```python
from build123d import *

# Parameters (mm, degrees)
CUT_EXTRUDE1_DEPTH   = 4.953
MIRROR2_COPY_1_DEPTH = 4.953
LPATTERN1_COUNT      = 4
LPATTERN1_PITCH      = 4.92125
SKETCH5_R            = 4.7625
CUT_EXTRUDE2_DEPTH   = 24.60625


with BuildPart() as part:
    # Sketch2 → Revolve1 (revolve)
    with BuildSketch(Plane(origin=(0, 0, 0), x_dir=(0, 0, -1), z_dir=(1, 0, 0))):
        Polygon((-55.5625, 0), (-55.5625, 7.46125), (-30.95625, 7.46125), (-30.95625, 14.2875), (30.95625, 14.2875), (30.95625, 7.46125), (55.5625, 7.46125), (55.5625, 0), align=None)
    revolve(axis=Axis((0, 0, -30.95625), (0, 0, 1)))

    # Sketch3 → Cut-Extrude1 (cut)
    with BuildSketch(Plane(origin=(0, 0, -30.95625), x_dir=(-1, 0, 0), z_dir=(0, 0, -1))):
        with BuildLine():
            Line((-8.5725, 11.43), (8.5725, 11.43))
            ThreePointArc((8.5725, 11.43), (0, 14.2875), (-8.5725, 11.43))
        make_face()
    cut_extrude1 = extrude(amount=-CUT_EXTRUDE1_DEPTH, mode=Mode.SUBTRACT)

    # Mirror1: Cut-Extrude1 across plane
    add(cut_extrude1.mirror(Plane.ZX), mode=Mode.SUBTRACT)

    # Mirror2: Cut-Extrude1 across plane
    add(cut_extrude1.mirror(Plane.XY), mode=Mode.SUBTRACT)

    # Mirror2 copy 1 sketch → Mirror2 copy 1 (cut)
    with BuildSketch(Plane(origin=(0, 0, 30.95625), x_dir=(-1, 0, 0), z_dir=(0, 0, 1))):
        with BuildLine():
            Line((-8.5725, 11.43), (8.5725, 11.43))
            ThreePointArc((8.5725, 11.43), (0, 14.2875), (-8.5725, 11.43))
        make_face()
    extrude(amount=-MIRROR2_COPY_1_DEPTH, mode=Mode.SUBTRACT)

    # Sketch4 → Cut-Revolve1 (revolve, cut)
    with BuildSketch(Plane(origin=(0, 0, 0), x_dir=(0, 0, -1), z_dir=(1, 0, 0))):
        Polygon((-55.5625, 7.46125), (-55.5625, 6.35), (-50.64125, 7.46125), align=None)
    cut_revolve1 = revolve(axis=Axis((0, 0, -55.5625), (0, 0, 1)), mode=Mode.SUBTRACT)

    # LPattern1: Cut-Revolve1 ×4
    with Locations(*[(0, 0, -i * LPATTERN1_PITCH) for i in range(1, LPATTERN1_COUNT)]):
        add(cut_revolve1, mode=Mode.SUBTRACT)

    # Mirror3: Cut-Revolve1 across plane
    add(cut_revolve1.mirror(Plane.XY), mode=Mode.SUBTRACT)

    # Mirror3 copy 1 sketch → Mirror3 copy 1 (revolve, cut)
    with BuildSketch(Plane(origin=(0, 0, 4.92125), x_dir=(0, 0, 1), z_dir=(1, 0, 0))):
        Polygon((-55.5625, -7.46125), (-55.5625, -6.35), (-50.64125, -7.46125), align=None)
    revolve(axis=Axis((0, 0, 60.48375), (0, 0, 1)), mode=Mode.SUBTRACT)

    # Mirror3 copy 2 sketch → Mirror3 copy 2 (revolve, cut)
    with BuildSketch(Plane(origin=(0, 0, 9.8425), x_dir=(0, 0, 1), z_dir=(1, 0, 0))):
        Polygon((-55.5625, -7.46125), (-55.5625, -6.35), (-50.64125, -7.46125), align=None)
    revolve(axis=Axis((0, 0, 65.405), (0, 0, 1)), mode=Mode.SUBTRACT)

    # Mirror3 copy 3 sketch → Mirror3 copy 3 (revolve, cut)
    with BuildSketch(Plane(origin=(0, 0, 14.76375), x_dir=(0, 0, 1), z_dir=(1, 0, 0))):
        Polygon((-55.5625, -7.46125), (-55.5625, -6.35), (-50.64125, -7.46125), align=None)
    revolve(axis=Axis((0, 0, 70.32625), (0, 0, 1)), mode=Mode.SUBTRACT)

    # Sketch5 → Cut-Extrude2 (cut)
    with BuildSketch(Plane.XY.offset(55.5625)):
        Circle(SKETCH5_R)
    cut_extrude2 = extrude(amount=-CUT_EXTRUDE2_DEPTH, mode=Mode.SUBTRACT)

    # Mirror4: Cut-Extrude2 across plane
    add(cut_extrude2.mirror(Plane.XY), mode=Mode.SUBTRACT)


solid = part.part
```
The listing builds one solid part. Answer for the finished solid, in the listing's coordinates (mm). A direction names the side the tool comes from. Coordinates: 2 decimals unless noted, no trailing zeros. Write each loop counter-clockwise with the first axis right and the second up, starting at its lowest first coordinate (ties: lowest second). Pieces come first, ordered by that corner, then holes. Notation, with made-up numbers: M -26.75,-23 L 32.25,-23 A30 cw 32.25,13 Z; hole C -10.75,47 d10. An arc over 180 degrees is marked long. Use a Markdown table: item, result. Add a question column.
1. Section B-B (z = -14) is taken. Give the vertices of the cut face in (x, y) (1 decimal), plus the area to 3 significant figures.
2. For a pull along X with two mould halves and no side action, classify faces 5 (the flat face through (0, -8, -30.956)), 6 (the flat face through (0, 0, 30.956)), 7 (the conical face through (6.387, -1.418, -54.708)) as +X half, -X half, draft (parallel to the pull), parting line (faces both ways), or undercut.
3. Section C-C (y = 8.5) is taken. Give the vertices of the cut face in (x, z), plus the area to 3 significant figures.
4. Straight lines are drawn through the part: line 1 along Z through (x, y) = (10, 4); line 2 along Z through (x, y) = (3, -12.25); line 3 along Y through (x, z) = (0, 44.75). For each, find the intervals that lie inside material, in ascending order. Write a range as [from, to].
5. Section A-A (z = 34) is taken. Give the vertices of the cut face in (x, y) (1 decimal), plus the area to 3 significant figures.
6. Given P1, Ø1.5, axis at x = 2.5, z = 29.5, coming from the -Y side; P2, Ø4, axis at y = -10, z = 1.5, coming from the -X side; P3, Ø2.5, axis at x = 0.5, y = 12.5, coming from the +Z side; P4, Ø2, axis at y = 10, z = -32.5, coming from the +X side, each flat-ended and moving along its own axis, determine where each tip first touches the part or whether it passes through.
7. Which of the six approach directions +Z, -Z, +X, -X, +Y, -Y give full straight-line access (tool end or side, diameter ignored) to faces 1 (the flat face through (0, -13, -26.003)), 2 (the cylindrical face through (-3.78, -2.9, -43.43)), 3 (the conical face through (6.387, -1.418, -44.865)), 4 (the flat face through (0, 13, 26.003))?
8. Section D-D (x = -11.5) is taken. Give the vertices of the cut face in (y, z).
Data:
| question | item | result |
|---|---|---|
| 1 | outline | C 0,0 d28.6 |
| 1 | area | 641 mm2 |
| 2 | face 5 | draft |
| 2 | face 6 | undercut |
| 2 | face 7 | parting line |
| 3 | outline | M -11.48,-30.96 L 11.48,-30.96 L 11.48,30.96 L -11.48,30.96 Z |
| 3 | area | 1,420 mm2 |
| 4 | line 1 | z = [-30.96, 30.96] |
| 4 | line 2 | z = [-26, 26] |
| 4 | line 3 | y = [-6.57, -4.76], [4.76, 6.57] |
| 5 | outline | C 0,0 d14.9; hole C 0,0 d9.5 |
| 5 | area | 104 mm2 |
| 6 | P1 | stops at y = -11.43 |
| 6 | P2 | stops at x = -11.84 |
| 6 | P3 | stops at z = 30.96 |
| 6 | P4 | passes through |
| 7 | face 1 | -Z, +X, -X, -Y |
| 7 | face 2 | -Z |
| 7 | face 3 | none |
| 7 | face 4 | +Z, +X, -X, +Y |
| 8 | outline | M -8.48,-30.96 L 8.48,-30.96 L 8.48,30.96 L -8.48,30.96 Z |
